Source: CAD feature listing. Evaluate the final solid. Frame: model axes, mm. Face numbers are marked on the shaded views. A direction names the side the tool comes from. Coordinates: 2 decimals unless noted, no trailing zeros. Loops run counter-clockwise (first coordinate to the right, second up) from the corner with the lowest first, then second, coordinate; pieces in that order, holes last.
from build123d import *

# Parameters (mm, degrees)
BOSS_EXTRUDE1_DEPTH = 65
CHAMFER1_SIZE       = 6
BOSS_EXTRUDE2_DEPTH = 2.5
SKETCH3_R           = 19.05
SKETCH3_R_2         = 2.75
CUT_EXTRUDE1_DEPTH  = 3
CUT_EXTRUDE2_DEPTH  = 3


with BuildPart() as part:
    # Sketch1 → Boss-Extrude1 (new body)
    with BuildSketch(Plane.XY):
        Polygon((0, 0), (0, 68), (3, 68), (3, 3), (68, 3), (68, 0), align=None)
    extrude(amount=BOSS_EXTRUDE1_DEPTH)

    # Chamfer1
    chamfer1_edges = [part.edges().sort_by_distance(p)[0] for p in [
        (1.5, 68, 65),
        (1.5, 68, 0),
        (68, 1.5, 65),
        (68, 1.5, 0),
    ]]
    chamfer(chamfer1_edges, length=CHAMFER1_SIZE)

    # Sketch2 → Boss-Extrude2 (add)
    with BuildSketch(Plane.XY.offset(65)):
        Polygon((4.600185007, 23.955878092), (23.955878092, 4.600185007), (23.955878092, 3), (7.047822016, 3), (3, 7.047822016), (3, 23.955878092), align=None)
    boss_extrude2 = extrude(amount=-BOSS_EXTRUDE2_DEPTH)

    # Mirror1: Boss-Extrude2 across plane
    add(boss_extrude2.mirror(Plane.XY.offset(32.5)))

    # Sketch3 → Cut-Extrude1 (cut)
    with BuildSketch(Plane.ZY):
        with Locations((32.5, 39)):
            Circle(SKETCH3_R)
        with Locations((8.95, 62.55)):
            Circle(SKETCH3_R_2)
        with Locations((56.05, 62.55)):
            Circle(SKETCH3_R_2)
        with Locations((8.95, 15.45)):
            Circle(SKETCH3_R_2)
        with Locations((56.05, 15.45)):
            Circle(SKETCH3_R_2)
    extrude(amount=-CUT_EXTRUDE1_DEPTH, mode=Mode.SUBTRACT)

    # Sketch4 → Cut-Extrude2 (cut)
    with BuildSketch(Plane.XZ):
        with BuildLine():
            Line((16.1, 54.65), (57.8, 54.65))
            ThreePointArc((57.8, 54.65), (59.95, 52.5), (57.8, 50.35))
            Line((57.8, 50.35), (16.1, 50.35))
            ThreePointArc((16.1, 50.35), (13.95, 52.5), (16.1, 54.65))
        make_face()
        with BuildLine():
            Line((16.1, 14.65), (57.8, 14.65))
            ThreePointArc((57.8, 14.65), (59.95, 12.5), (57.8, 10.35))
            Line((57.8, 10.35), (16.1, 10.35))
            ThreePointArc((16.1, 10.35), (13.95, 12.5), (16.1, 14.65))
        make_face()
    extrude(amount=-CUT_EXTRUDE2_DEPTH, mode=Mode.SUBTRACT)


solid = part.part
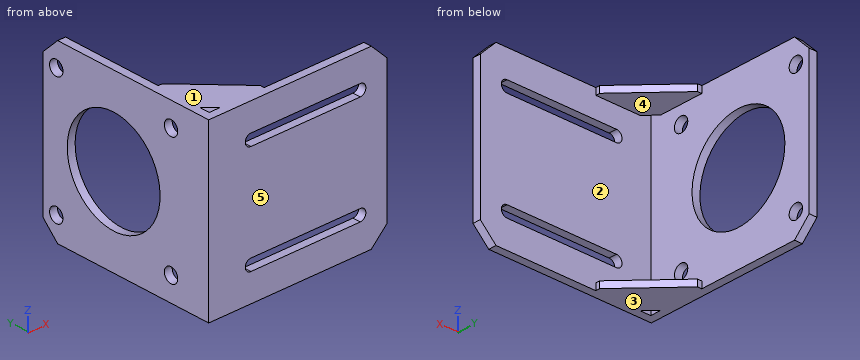
Q1. Line query: line 1 along Y through (x, z) = (1, 56); line 2 along Y through (x, z) = (9.5, 4.5); line 3 along Y through (x, z) = (2, 8). Output: solid intervals per line, ascending.
Q2. Section B-B, the plane y = 39. Return the cut outline in (x, z).
Q3. Contact query for flat-ended pins moving along their axis: pin 1 Ø2 at (y, z) = (18, 22) entering from +X; pin 2 Ø5 at (x, z) = (57, 31) entering from +Y; pin 3 Ø0.8 at (x, z) = (4, 63.5) entering from +Y. Output: stop coordinate, or through.
Q4. Section C-C, the plane z = 32.5. Return the cut outline in (x, y), plus the area to 3 significant figures.
Q5. Access query for the marked faces 4 and 5. Directions: +Z, -Z, +X, -X, +Y, -Y. A direction counts if a zero-diameter tool reaches every point of the face in a straight line with its end or side. Return the directions, or none.
Q6. Section A-A, the plane z = 56.05. Return the cut outline in (x, y).
Q7. Draft query along Z for the marked faces 1, 2 and 3. Return one class per face: +Z half, -Z half, draft (parallel to the pull), parting line (faces both ways), or undercut.
Q8. Section D-D, the plane x = 15. Return the cut outline in (y, z).
Derived:
1. line 1: y = 0 to 12.7, 18.2 to 59.8, 65.3 to 68
1. line 2: y = 0 to 3
1. line 3: y = 0 to 12.87, 18.03 to 59.97, 65.13 to 68
2. outline: (0, 0) - (3, 0) - (3, 13.45) - (0, 13.45) - close; (0, 51.55) - (3, 51.55) - (3, 65) - (0, 65) - close
3. pin 1: stops at x = 3
3. pin 2: stops at y = 3
3. pin 3: stops at y = 23.96
4. outline: (0, 0) - (68, 0) - (68, 3) - (3, 3) - (3, 19.95) - (0, 19.95) - close; (0, 58.05) - (3, 58.05) - (3, 68) - (0, 68) - close
4. area: 285 mm2
5. face 4: +X, +Y
5. face 5: +Z, -Z, +X, -X, -Y
6. outline: (0, 0) - (68, 0) - (68, 3) - (3, 3) - (3, 12.7) - (0, 12.7) - close; (0, 18.2) - (3, 18.2) - (3, 59.8) - (0, 59.8) - close; (0, 65.3) - (3, 65.3) - (3, 68) - (0, 68) - close
7. face 1: +Z half
7. face 2: undercut
7. face 3: -Z half
8. outline: (0, 0) - (13.56, 0) - (13.56, 2.5) - (3, 2.5) - (3, 10.65) - (0, 10.65) - close; (0, 14.35) - (3, 14.35) - (3, 50.65) - (0, 50.65) - close; (0, 54.35) - (3, 54.35) - (3, 62.5) - (13.56, 62.5) - (13.56, 65) - (0, 65) - close
